Autodesk Inventor part; units mm, degrees
ref_plane "YZ Plane" through (0, 0, 0) normal (1, 0, 0) x (0, 1, 0)
ref_plane "XZ Plane" through (0, 0, 0) normal (0, 1, 0) x (-1, 0, 0)
ref_plane "XY Plane" through (0, 0, 0) normal (0, 0, 1) x (1, 0, 0)
sketch "スケッチ1" plane through (0, 0, 0) normal (0, 0, 1) x (1, 0, 0)
  circle A0 centre (0, 0) radius 6.2
  line L0 (-9, 0) -> (9, 0) construction
  circle A1 centre (9, 0) radius 1.6
  circle A2 centre (-9, 0) radius 1.6
  line L1 (15, 10) -> (-15, 10) construction
  circle A3 centre (15, 10) radius 1.6
  circle A4 centre (-15, 10) radius 1.6
  arc A5 (-6.1356, 0.8916) -> (-6.1356, -0.8916) centre (-9, 0) ccw
  arc A6 (6.1356, -0.8916) -> (6.1356, 0.8916) centre (9, 0) ccw
  line L2 (17.5725, 8.4565) -> (11.5725, -1.5435)
  line L3 (11, -2.2361) -> (6, -6.7082)
  line L4 (-6, -6.7082) -> (-11, -2.2361)
  line L5 (-11.5725, -1.5435) -> (-17.5725, 8.4565)
  arc A7 (-13.5062, 12.6017) -> (13.5062, 12.6017) centre (0, 36.125) ccw
  arc A8 (-8.5, -2.958) -> (8.5, -2.958) centre (0, 0) ccw
  arc A9 (-12.3272, 8.6376) -> (-6.0941, 6.6228) centre (0, 36.125) ccw
  arc A10 (6.0941, 6.6228) -> (12.3272, 8.6376) centre (0, 36.125) ccw
  line L6 (-10.5435, 2.5725) -> (-13.4565, 7.4275)
  line L7 (13.4565, 7.4275) -> (10.5435, 2.5725)
  arc A11 (8.5, 2.958) -> (6.0941, 6.6228) centre (0, 0) ccw
  arc A12 (-6.0941, 6.6228) -> (-8.5, 2.958) centre (0, 0) ccw
  arc A13 (-13.5062, 12.6017) -> (-17.5725, 8.4565) centre (-15, 10) ccw
  arc A14 (-13.4565, 7.4275) -> (-12.3272, 8.6376) centre (-15, 10) ccw
  arc A15 (17.5725, 8.4565) -> (13.5062, 12.6017) centre (15, 10) ccw
  arc A16 (12.3272, 8.6376) -> (13.4565, 7.4275) centre (15, 10) ccw
  point P0 (0, 10)
  dimension "d0" = 12.4
  dimension "d1" = 18
  dimension "d2" = 3.2
  dimension "d3" = 3.2
  dimension "d4" = 3.2
  dimension "d5" = 3.2
  dimension "d6" = 10
  dimension "d7" = 30
  dimension "d10" = 6
  dimension "d11" = 6
  dimension "d13" = 9
  dimension "d15" = 3
  dimension "d18" = 3
  dimension "d20" = 3
  dimension "d21" = 3
extrude "押し出し1" add sketch "スケッチ1" along normal blind 3 contours A0 A6 | A0 A5 A12 A9 A14 L6 L5 A13 A7 A15 L2 A6 L7 A16 A10 A11 | A6 A8 A5 A0 | A0 A5 | A6 L3 A8 | A8 L4 A5
properties part number "EncoderMount"
Can you work these out from the model? Positions are in its coordinate system, mm. A direction names the side the tool comes from. Coordinates: 2 decimals unless noted, no trailing zeros. Loops run counter-clockwise (first coordinate to the right, second up) from the corner with the lowest first, then second, coordinate; pieces in that order, holes last. Notation, with made-up numbers: M 55.5,-22 L 63.5,-22 A22 cw 63.5,0 Z; hole C -30,-36.75 d11. An arc over 180 degrees is marked long. Answer as CSV lines item,"result". Start each with the question number.
1. Suppose I cut it at A-A, the plane x = 0. List the corners of the cut face in (y, z) for me.
2. Suppose I cut it at C-C, the plane z = 0.4. List the corners of the cut face in (x, y) for me (1 decimal).
3. Suppose I cut it at D-D, the plane y = -5. List the corners of the cut face in (x, z) for me, plus the area to 3 significant figures.
4. Suppose I cut it at B-B, the plane x = -9. List the corners of the cut face in (y, z) for me, plus the area to 3 significant figures.
5. Thinking about a two-plate mould opening in Y: for faces 3 (the face through (-16.27, 10.97, 1.48)), 4 (the face through (-8.47, -4.5, 1.48)), 5 (the face through (-17.18, 12.06, 1.48)), which applies, +Y half, -Y half, draft (parallel to the pull), parting line (faces both ways), or undercut?
6. For faces 1 (the face through (0, 7, 0)), 2 (the face through (9.54, 2.95, 1.48)), which set-ups out of +Z, -Z, +X, -X, +Y, -Y let a thin tool reach every point of the face, with its end or its side?
7. If I drill on probe 1 along Y at (x, z) = (0, 2.4); probe 2 along Y at (x, z) = (-9, 0.9); probe 3 along X at (y, z) = (4.5, 1.75), over which ranges is the centre line in solid material (lowest first)? Write a range as [from, to].
8. For pin 1 Ø1.5 at (y, z) = (-6, 2) entering from +X, with a flat end and sliding along its axis, tell me the tip position at first contact or that it passes through.
Output:
1,outline,"M -9,0 L -6.2,0 L -6.2,3 L -9,3 Z; M 6.2,0 L 9,0 L 9,3 L 6.2,3 Z"
2,outline,"M -17.6,8.5 L -11.6,-1.5 A3 ccw -11,-2.2 L -6,-6.7 A9 ccw 6,-6.7 L 11,-2.2 A3 ccw 11.6,-1.5 L 17.6,8.5 A3 ccw 13.5,12.6 A27.1 cw -13.5,12.6 A3 ccw Z; hole C -15,10 d3.2; hole M -13.5,7.4 L -10.5,2.6 A3 cw -8.5,3 A9 cw -6.1,6.6 A30.1 cw -12.3,8.6 A3 cw Z; hole C -9,0 d3.2; hole C 0,0 d12.4; hole M 6.1,6.6 A9 cw 8.5,3 A3 cw 10.5,2.6 L 13.5,7.4 A3 cw 12.3,8.6 A30.1 cw Z; hole C 9,0 d3.2; hole C 15,10 d3.2"
3,outline,"M -7.91,0 L -3.67,0 L -3.67,3 L -7.91,3 Z; M 3.67,0 L 7.91,0 L 7.91,3 L 3.67,3 Z"
3,area,"25.5 mm^2"
4,outline,"M -4.02,0 L -1.6,0 L -1.6,3 L -4.02,3 Z; M 1.6,0 L 3,0 L 3,3 L 1.6,3 Z; M 7.38,0 L 10.54,0 L 10.54,3 L 7.38,3 Z"
4,area,"21.0 mm^2"
5,face 3,"undercut"
5,face 4,"-Y half"
5,face 5,"parting line"
6,face 1,"-Z, +X, -X, +Y, -Y"
6,face 2,"+Z, -Z"
7,probe 1,"y = [-9, -6.2], [6.2, 9]"
7,probe 2,"y = [-4.02, -1.6], [1.6, 3], [7.38, 10.54]"
7,probe 3,"x = [-15.2, -11.7], [-7.79, -4.26], [4.26, 7.79], [11.7, 15.2]"
8,pin 1,"stops at x = 7.63"
